from build123d import *

# Parameters (mm, degrees)
CUT_EXTRUDE1_DEPTH = 1.1


with BuildPart() as part:
    # Sketch1 → Revolve1 (revolve)
    with BuildSketch(Plane.XY, mode=Mode.PRIVATE) as revolve1_sk:
        Polygon((0, 0.672649731), (1, 1.25), (1, 2.195299462), (1.154700538, 2.35), (2, 2.35), (2.25, 2.1), (2.25, 0.0625), (2.1875, 0), (1.3, 0), (1.25, -0.51), (1.25, -7.724), (0.974, -8), (0, -8), align=None)
    revolve(revolve1_sk.sketch.rotate(Axis((0, -8, 0), (0, 1, 0)), 270), axis=Axis((0, -8, 0), (0, 1, 0)))

    # Sketch2 → Cut-Extrude1 (cut)
    with BuildSketch(Plane(origin=(0, 2.35, 0), x_dir=(1, 0, 0), z_dir=(0, 1, 0))):
        Polygon((-1, -0.577350269), (0, -1.154700538), (1, -0.577350269), (1, 0.577350269), (0, 1.154700538), (-1, 0.577350269), align=None)
    extrude(amount=-CUT_EXTRUDE1_DEPTH, mode=Mode.SUBTRACT)


solid = part.part
Model file for the job. Use its own axes, mm. A direction names the side the tool comes from. Give positions to 0.01 mm unless a question says otherwise; leave off trailing zeros. Order: outer loops, then holes, each group sorted by start corner. A loop starts at its lowest first (then second) coordinate and runs counter-clockwise, first axis right, second up. Notation, with made-up numbers: M 76,9 L 91,9 A37 ccw 91,46 Z; hole C 55,6.5 d9. An arc over 180 degrees is marked long. Put each result on its own line as item: value. Start each with the question number.
(1) Pin check, flat tips, straight feed: pin 1 Ø1 at (y, z) = (-5, -1) entering from +X; pin 2 Ø1 at (x, y) = (-0.5, -1.5) entering from -Z; pin 3 Ø1.5 at (x, y) = (-0.5, -5.5) entering from +Z. Stop position of each tip, or through.
(2) Drill centre lines: L1, parallel to Z at x = -0.05, y = -2.25; L2, parallel to Z at x = -0.75, y = -5; L3, parallel to Y at x = 1.65, z = 0.55. Where is each one in solid material? Low to high. Write a range as [from, to].
(3) Band-saw the part on B-B on y = 1. Give the cut face in (x, z), then the cut area to 3 significant figures.
(4) Pull direction X, two halves, no side cores. Call faces 4 (the face through (-1, 2.35, -1)), 5 (the face through (-0.49, 1.81, -0.87)), 6 (the face through (0.676, 1.067, 2.146)): released by +X, released by -X, zero draft, split by the parting line, or undercut.
(5) Band-saw the part on A-A on y = -5.25. Give the cut face in (x, z), then the cut area to 3 significant figures.
(6) Tool access for faces 1 (the face through (0, -8, 0)), 2 (the face through (1, 2, 0)), 3 (the face through (-1.4, 0, 0.5)): list every direction of +Z, -Z, +X, -X, +Y, -Y with a clear straight run to the whole face (end or side of a thin tool).
Results below:
1. pin 1: stops at x = 1.15
1. pin 2: stops at z = -1.25
1. pin 3: stops at z = 1.25
2. L1: z = [-1.25, 1.25]
2. L2: z = [-1, 1]
2. L3: y = [0, 2.35]
3. outline: C 0,0 d4.5; hole C 0,0 d1.13
3. area: 14.9 mm2
4. face 4: zero draft
4. face 5: undercut
4. face 6: split by the parting line
5. outline: C 0,0 d2.5
5. area: 4.91 mm2
6. face 1: +Z, -Z, +X, -X, -Y
6. face 2: +Y
6. face 3: -Y
